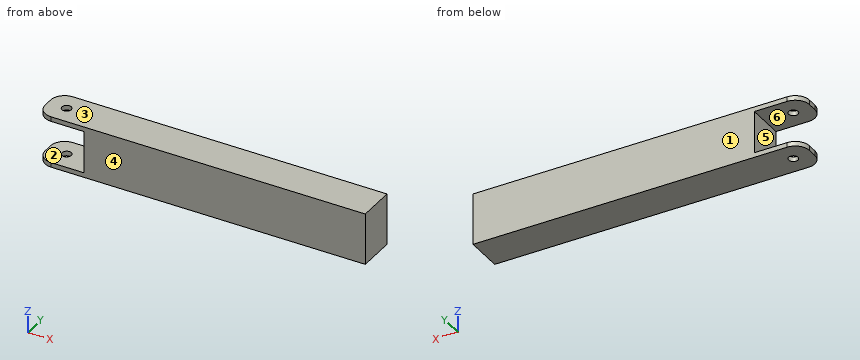
```python
from build123d import *

# Parameters (mm, degrees)
SKETCH1_W            = 300
SKETCH1_H            = 40
BOSS_EXTRUDE1_DEPTH  = 22.5
SKETCH2_W            = 350
SKETCH2_H            = 40
SKETCH2_R            = 5
BOSS_EXTRUDE2_DEPTH  = 5
FILLET1_R            = 15
FILLET1_OF_MIRROR1_R = 15


with BuildPart() as part:
    # Sketch1 → Boss-Extrude1 (new, symmetric)
    with BuildSketch(Plane.XY):
        Rectangle(SKETCH1_W, SKETCH1_H)
    extrude(amount=BOSS_EXTRUDE1_DEPTH, both=True)

    # Sketch2 → Boss-Extrude2 (add)
    with BuildSketch(Plane.XY.offset(22.5)):
        with Locations((-25, 0)):
            Rectangle(SKETCH2_W, SKETCH2_H)
        with Locations((-180, 0)):
            Circle(SKETCH2_R, mode=Mode.SUBTRACT)
    boss_extrude2 = extrude(amount=BOSS_EXTRUDE2_DEPTH)

    # Fillet1
    fillet1_edges = [part.edges().sort_by_distance(p)[0] for p in [
        (-200, -20, 25),
        (-200, 20, 25),
    ]]
    fillet(fillet1_edges, radius=FILLET1_R)

    # Mirror1: Boss-Extrude2 across plane
    add(boss_extrude2.mirror(Plane.XY))

    # Fillet1 of Mirror1
    fillet1_of_mirror1_edges = [part.edges().sort_by_distance(p)[0] for p in [
        (-200, -20, -25),
        (-200, 20, -25),
    ]]
    fillet(fillet1_of_mirror1_edges, radius=FILLET1_OF_MIRROR1_R)


solid = part.part
```
Can you work these out from the model? Positions are in its coordinate system, mm. Face numbers are marked on the shaded views. A direction names the side the tool comes from. Round coordinates to 2 decimals unless told otherwise and drop trailing zeros. Loops run counter-clockwise (first coordinate to the right, second up) from the corner with the lowest first, then second, coordinate; pieces in that order, holes last. Notation, with made-up numbers: M 32,60 L 55,60 A15 cw 55,89 Z; hole C 19.5,1.5 d4. An arc over 180 degrees is marked long. Answer in a Markdown table with one row per item.
1. On a 3-axis mill with a long thin cutter (end or side, diameter ignored), from which of +Z, -Z, +X, -X, +Y, -Y can I reach the whole of each face in a straight line? I mean the marked faces 1 and 2. Say none if no direction works.
Established:
| item | result |
|---|---|
| face 1 | +Z, -Z, +X, -X, +Y |
| face 2 | -X, +Y, -Y |
2. Please list where these lines run through material, in increasing order: line 1 (Y direction, x = -180, z = 25); line 2 (Z direction, x = -158, y = -8); line 3 (X direction, y = -10.5, z = 8.5). Write a range as from..to.
Established:
| item | result |
|---|---|
| line 1 | -20..-5, 5..20 |
| line 2 | -27.5..-22.5, 22.5..27.5 |
| line 3 | -150..150 |
3. Thinking about a two-plate mould opening in Z: for the marked faces 3, 4, 5 and 6, which applies, pulls with the +Z half, pulls with the -Z half, needs draft (parallel to the pull), parting line crosses it, or undercut?
Established:
| item | result |
|---|---|
| face 3 | pulls with the +Z half |
| face 4 | needs draft |
| face 5 | undercut |
| face 6 | undercut |
4. If we section it at C-C, the plane z = 4: Please give me the cut outline in (x, y), plus the area to 3 significant figures.
Established:
| item | result |
|---|---|
| outline | M -150,-20 L 150,-20 L 150,20 L -150,20 Z |
| area | 12,000 mm² |
5. I'm going to push a flat-ended pin straight in: pin 1 Ø3 at (y, z) = (-10, 9) entering from -X. Where does the tip first touch, or does it pass through?
Established:
| item | result |
|---|---|
| pin 1 | x = -150 |
6. If we section it at B-B, the plane y = 0: Please give me the cut outline in (x, z), plus the area to 3 significant figures.
Established:
| item | result |
|---|---|
| outline | M -200,-27.5 L -185,-27.5 L -185,-22.5 L -200,-22.5 Z; M -200,22.5 L -185,22.5 L -185,27.5 L -200,27.5 Z; M -175,-27.5 L 150,-27.5 L 150,27.5 L -175,27.5 L -175,22.5 L -150,22.5 L -150,-22.5 L -175,-22.5 Z |
| area | 16,900 mm² |
7. If we section it at A-A, the plane x = -180: Please give me the cut outline in (y, z).
Established:
| item | result |
|---|---|
| outline | M -20,-27.5 L -5,-27.5 L -5,-22.5 L -20,-22.5 Z; M -20,22.5 L -5,22.5 L -5,27.5 L -20,27.5 Z; M 5,-27.5 L 20,-27.5 L 20,-22.5 L 5,-22.5 Z; M 5,22.5 L 20,22.5 L 20,27.5 L 5,27.5 Z |
